Design review of the part built by this model. Coordinates are the model's own, in mm. A direction names the side the tool comes from. Give positions to 0.01 mm unless a question says otherwise; leave off trailing zeros. Write each loop counter-clockwise with the first axis right and the second up, starting at its lowest first coordinate (ties: lowest second). Pieces come first, ordered by that corner, then holes. Notation, with made-up numbers: (20.5, 20) -> (24.5, 20) arc R18 cw to (24.5, 29) -> close; hole circle Ø11 at (15.25, -26). An arc over 180 degrees is marked (long way). Write each question's results on one line, items separated by ' | '. Start each with the question number.
(1) For faces 5 (the face through (0, 1, -42)), 6 (the face through (39.5, 1, -14)), 7 (the face through (0.4, 4, -28)), 8 (the face through (20, 2, -54.5)), 9 (the face through (0, 1, -14)), list the 3-axis set-ups (+Z, -Z, +X, -X, +Y, -Y) from which the entire face can be reached by the end or side of a thin tool; tool diameter is ignored.
(2) To check wall thickness, follow probe 1 along X at (y, z) = (2.75, -36); probe 2 along Z at (x, y) = (18.5, 4); probe 3 along Z at (x, y) = (36, 2.55). State the ranges of each line that lie inside material, in increasing order.
(3) Take a section at A-A (y = 5.3). State the section outline as (x, z) points, plus the area to 3 significant figures.
(4) Take a section at C-C (z = -50). State the section outline as (x, y) points, plus the area to 4 significant figures.
(5) Take a section at D-D (x = 4). State the section outline as (y, z) points, plus the area to 3 significant figures.
(6) Take a section at B-B (x = 20). State the section outline as (y, z) points.
(7) Mouldability with a two-part tool opening along Z and no side actions: class faces 1 (the face through (10, 1, 0)), 2 (the face through (20, 6, -57)), 3 (the face through (20, 4, -0.4)), 4 (the face through (20, 2, -1.5)) as released by +Z, released by -Z, zero draft, split by the parting line, or undercut.
(8) Clearance check with flat-ended pins moving along their axes: pin 1 (0.6 mm diameter, centred on y = 4.5, z = -56.5, fed in from +X); pin 2 (1.5 mm diameter, centred on x = 12.5, y = 2, fed in from -Z); pin 3 (0.6 mm diameter, centred on x = -0.5, y = 2, fed in from +Z). State where each tip first meets the part, or that it passes through.
from build123d import *

# Parameters (mm, degrees)
SKETCH1_W           = 39.5
SKETCH1_H           = 56
BOSS_EXTRUDE1_DEPTH = 3
FILLET1_R           = 3
SHELL1_T            = -1.5
SKETCH2_W           = 5
SKETCH2_H           = 3
BOSS_EXTRUDE2_DEPTH = 1.5
SKETCH3_W           = 1.9
SKETCH3_H           = 5
BOSS_EXTRUDE3_DEPTH = 3
SKETCH8_W           = 5
SKETCH8_H           = 3
BOSS_EXTRUDE5_DEPTH = 1.5
SKETCH9_W           = 5
SKETCH9_H           = 1.9
BOSS_EXTRUDE6_DEPTH = 3


with BuildPart() as part:
    # Sketch1 → Boss-Extrude1 (new body)
    with BuildSketch(Plane(origin=(0, 0, 0), x_dir=(1, 0, 0), z_dir=(0, 1, 0))):
        with Locations((19.75, 28)):
            Rectangle(SKETCH1_W, SKETCH1_H)
    extrude(amount=BOSS_EXTRUDE1_DEPTH)

    # Fillet1
    fillet1_edges = [part.edges().sort_by_distance(p)[0] for p in [
        (0, 1.5, -56),
        (39.5, 1.5, -56),
        (39.5, 1.5, 0),
        (0, 1.5, 0),
    ]]
    fillet(fillet1_edges, radius=FILLET1_R)

    # Shell1
    shell1_openings = [part.faces().sort_by_distance(p)[0] for p in [
        (19.75, 3, -28),
    ]]
    offset(amount=SHELL1_T, openings=shell1_openings, kind=Kind.INTERSECTION)

    # Sketch2 → Boss-Extrude2 (add)
    with BuildSketch(Plane.ZY):
        with Locations((-28.5, 1.5)):
            Rectangle(SKETCH2_W, SKETCH2_H)
    boss_extrude2 = extrude(amount=BOSS_EXTRUDE2_DEPTH)

    # Sketch3 → Boss-Extrude3 (add)
    with BuildSketch(Plane(origin=(0, 3, 0), x_dir=(1, 0, 0), z_dir=(0, 1, 0))):
        with Locations((-0.55, 28.5)):
            Rectangle(SKETCH3_W, SKETCH3_H)
    boss_extrude3 = extrude(amount=BOSS_EXTRUDE3_DEPTH)

    # Sketch8 → Boss-Extrude5 (add)
    with BuildSketch(Plane.XY):
        with Locations((19.75, 1.5)):
            Rectangle(SKETCH8_W, SKETCH8_H)
    boss_extrude5 = extrude(amount=BOSS_EXTRUDE5_DEPTH)

    # Sketch9 → Boss-Extrude6 (add)
    with BuildSketch(Plane(origin=(0, 3, 0), x_dir=(1, 0, 0), z_dir=(0, 1, 0))):
        with Locations((19.75, -0.55)):
            Rectangle(SKETCH9_W, SKETCH9_H)
    boss_extrude6 = extrude(amount=BOSS_EXTRUDE6_DEPTH)

    # Mirror3: Boss-Extrude2, Boss-Extrude3 across plane
    add(boss_extrude2.mirror(Plane(origin=(19.75, 0, 0), x_dir=(0, 0, 1), z_dir=(1, 0, 0))))
    add(boss_extrude3.mirror(Plane(origin=(19.75, 0, 0), x_dir=(0, 0, 1), z_dir=(1, 0, 0))))

    # Mirror4: Boss-Extrude5, Boss-Extrude6 across plane
    add(boss_extrude5.mirror(Plane(origin=(0, 0, -28), x_dir=(1, 0, 0), z_dir=(0, 0, -1))))
    add(boss_extrude6.mirror(Plane(origin=(0, 0, -28), x_dir=(1, 0, 0), z_dir=(0, 0, -1))))


solid = part.part
Report:
1) face 5: -Z, -X, +Y, -Y | face 6: +Z, +X, +Y, -Y | face 7: +Z, -Z, +Y | face 8: +Y | face 9: +Z, -X, +Y, -Y
2) probe 1: 0 to 1.5, 38 to 39.5 | probe 2: -57.5 to -55.6, -0.4 to 1.5 | probe 3: -56 to -54.5, -1.5 to 0
3) outline: (-1.5, -31) -> (0.4, -31) -> (0.4, -26) -> (-1.5, -26) -> close; (17.25, -57.5) -> (22.25, -57.5) -> (22.25, -55.6) -> (17.25, -55.6) -> close; (17.25, -0.4) -> (22.25, -0.4) -> (22.25, 1.5) -> (17.25, 1.5) -> close; (39.1, -31) -> (41, -31) -> (41, -26) -> (39.1, -26) -> close | area: 38.0 mm2
4) outline: (0, 0) -> (39.5, 0) -> (39.5, 3) -> (38, 3) -> (38, 1.5) -> (1.5, 1.5) -> (1.5, 3) -> (0, 3) -> close | area: 63.75 mm2
5) outline: (0, -56) -> (3, -56) -> (3, -54.5) -> (1.5, -54.5) -> (1.5, -1.5) -> (3, -1.5) -> (3, 0) -> (0, 0) -> close | area: 88.5 mm2
6) outline: (0, -57.5) -> (6, -57.5) -> (6, -55.6) -> (3, -55.6) -> (3, -54.5) -> (1.5, -54.5) -> (1.5, -1.5) -> (3, -1.5) -> (3, -0.4) -> (6, -0.4) -> (6, 1.5) -> (0, 1.5) -> close
7) face 1: released by +Z | face 2: zero draft | face 3: undercut | face 4: undercut
8) pin 1: x = 22.25 | pin 2: z = -56 | pin 3: z = -26
